from build123d import *

# Parameters (mm, degrees)
EXTRUDE_1_DEPTH     = 3
SKETCH_2_R          = 4
CUT_EXTRUDE_1_DEPTH = 8
SKETCH_3_R          = 1.5
CUT_EXTRUDE_2_DEPTH = 3
CUT_EXTRUDE_3_DEPTH = 10
FILLET_1_R          = 10
SKETCH_5_W          = 7.8
SKETCH_5_H          = 20.5
CUT_EXTRUDE_4_DEPTH = 10
FILLET_3_R          = 3


with BuildPart() as part:
    # 草图1 → 凸台-拉伸1 (new body)
    with BuildSketch(Plane(origin=(0, 0, 0), x_dir=(1, 0, 0), z_dir=(0, 1, 0))):
        with BuildLine():
            Line((-7.5, -29), (7.5, -29))
            Line((7.5, -29), (7.5, 29))
            ThreePointArc((7.5, 29), (0, 36.5), (-7.5, 29))
            Line((-7.5, 29), (-7.5, -29))
        make_face()
    extrude(amount=EXTRUDE_1_DEPTH)

    # 草图2 → 切除-拉伸1 (cut)
    with BuildSketch(Plane(origin=(0, 3, 0), x_dir=(1, 0, 0), z_dir=(0, 1, 0))):
        with Locations(Location((0, 29, 0), (0, 0, 270))):
            Circle(SKETCH_2_R)
    extrude(amount=-CUT_EXTRUDE_1_DEPTH, mode=Mode.SUBTRACT)

    # 草图3 → 切除-拉伸2 (cut)
    with BuildSketch(Plane.XZ):
        with Locations(Location((0, 1, 0), (0, 0, 270))):
            Circle(SKETCH_3_R)
        with Locations(Location((0, -9, 0), (0, 0, 270))):
            Circle(SKETCH_3_R)
    extrude(amount=-CUT_EXTRUDE_2_DEPTH, mode=Mode.SUBTRACT)

    # 草图4 → 切除-拉伸3 (cut)
    with BuildSketch(Plane.XZ):
        Polygon((-7.5, -13.5), (-3.9, -13.5), (-3.9, 26.5), (3.9, 26.5), (3.9, -13.5), (7.5, -13.5), (7.5, 29), (-7.5, 29), align=None)
    extrude(amount=-CUT_EXTRUDE_3_DEPTH, mode=Mode.SUBTRACT)

    # 圆角1
    # the kernel refuses this fillet: 10 mm, written as the material it takes off along each edge
    with BuildSketch(Plane(origin=(7.5, -19.209372712, -13.5), x_dir=(0, 0, -1), z_dir=(0, 1, 0))) as fillet_1_piece_1:
        with BuildLine():
            CenterArc((7.683749085, 10), FILLET_1_R, 219.7918195, 50.2081805)
            Line((0, 3.6), (-0.153674982, 3.472))
            ThreePointArc((-0.153674982, 3.472), (-0.2, 1.8), (-0.2, 0))
            Line((-0.2, 0), (0, -0.2))
            Line((0, -0.2), (7.683749085, -0.2))
            Line((7.683749085, -0.2), (7.683749085, 0))
        make_face()
    extrude(amount=41.418745425, mode=Mode.SUBTRACT)
    with BuildSketch(Plane(origin=(-7.5, -19.209372712, -13.5), x_dir=(0, 0, -1), z_dir=(0, 1, 0))) as fillet_1_piece_2:
        with BuildLine():
            CenterArc((7.683749085, -10), FILLET_1_R, 90, 50.2081805)
            Line((0, -3.6), (-0.153674982, -3.472))
            ThreePointArc((-0.153674982, -3.472), (-0.2, -1.8), (-0.2, 0))
            Line((-0.2, 0), (0, 0.2))
            Line((0, 0.2), (7.683749085, 0.2))
            Line((7.683749085, 0.2), (7.683749085, 0))
        make_face()
    extrude(amount=41.418745425, mode=Mode.SUBTRACT)

    # 草图5 → 切除-拉伸4 (cut)
    with BuildSketch(Plane(origin=(0, 3, 0), x_dir=(1, 0, 0), z_dir=(0, 1, 0))):
        with Locations((0, -16.25)):
            Rectangle(SKETCH_5_W, SKETCH_5_H)
    extrude(amount=-CUT_EXTRUDE_4_DEPTH, mode=Mode.SUBTRACT)

    # 圆角3
    fillet_3_edges = [part.edges().sort_by_distance(p)[0] for p in [
        (-3.9, 1.5, 6),
        (3.9, 1.5, 6),
    ]]
    fillet(fillet_3_edges, radius=FILLET_3_R)


solid = part.part
Model file for the job. Use its own axes, mm. A direction names the side the tool comes from. Give positions to 0.01 mm unless a question says otherwise; leave off trailing zeros. Loops run counter-clockwise (first coordinate to the right, second up) from the corner with the lowest first, then second, coordinate; pieces in that order, holes last. Notation, with made-up numbers: (68.25, 82.5) -> (119.25, 82.5) arc R16 ccw to (119.25, 112.5) -> close; hole circle Ø10 at (19.25, 28.25). An arc over 180 degrees is marked (long way). Use a Markdown table: item, result. Add a question column.
(1) Slice it at D-D on x = -6.5. List the corners of the cut face in (y, z), and give its area (3 significant figures).
(2) Wall check: line 1 along X through (y, z) = (2.3, 1); line 2 along X through (y, z) = (2.35, -29); line 3 along Z through (x, y) = (0.75, 2.3). Give the ranges that are in metal, low to high.
(3) Tool access for faces 1 (the flat face through (0, 3, -16)), 2 (the flat face through (3.9, 1, -5)): list every direction of +Z, -Z, +X, -X, +Y, -Y with a clear straight run to the whole face (end or side of a thin tool).
(4) Slice it at B-B on x = 0. List the corners of the cut face in (y, z), and give its area (3 significant figures).
(5) Slice it at C-C on y = 0.8. List the corners of the cut face in (x, z).
(6) Slice it at A-A on z = 1. List the corners of the cut face in (x, y).
(7) Mould opens along Z. For faces 3 (the flat face through (-3.9, 1, -5)), 4 (the cylindrical face through (1.01, 1.48, 2.11)), 5 (the cylindrical face through (-6.581, 1.479, -16.997)) say: +Z half, -Z half, draft (parallel to the pull), parting line (faces both ways), or undercut.
Filled sheet:
| question | item | result |
|---|---|---|
| 1 | outline | (0, -32.74) -> (3, -32.74) -> (3, -16.82) -> (0, -16.82) -> close |
| 1 | area | 47.8 mm2 |
| 2 | line 1 | -3.9 to -1.5, 1.5 to 3.9 |
| 2 | line 2 | -7.5 to -4, 4 to 7.5 |
| 2 | line 3 | -36.46 to -32.93, -25.07 to -10.3, -7.7 to -0.3, 2.3 to 6 |
| 3 | face 1 | +Z, -Z, +X, -X, +Y |
| 3 | face 2 | +Z, +X, +Y, -Y |
| 4 | outline | (0, -36.5) -> (3, -36.5) -> (3, -33) -> (0, -33) -> close; (0, -25) -> (3, -25) -> (3, -10.5) -> (0, -10.5) -> close; (0, -7.5) -> (3, -7.5) -> (3, -0.5) -> (0, -0.5) -> close; (0, 2.5) -> (3, 2.5) -> (3, 6) -> (0, 6) -> close |
| 4 | area | 85.5 mm2 |
| 5 | outline | (-7.5, -29) arc R7.5 ccw to (7.5, -29) -> (7.5, -21.18) arc R10 ccw to (3.9, -13.5) -> (3.9, 3) arc R3 ccw to (0.9, 6) -> (-0.9, 6) arc R3 ccw to (-3.9, 3) -> (-3.9, -13.5) arc R10 ccw to (-7.5, -21.18) -> close; hole circle Ø8 at (0, -29); hole circle Ø3 at (0, -9); hole circle Ø3 at (0, 1) |
| 6 | outline | (-3.9, 0) -> (-1.5, 0) -> (-1.5, 3) -> (-3.9, 3) -> close; (1.5, 0) -> (3.9, 0) -> (3.9, 3) -> (1.5, 3) -> close |
| 7 | face 3 | draft |
| 7 | face 4 | undercut |
| 7 | face 5 | +Z half |
